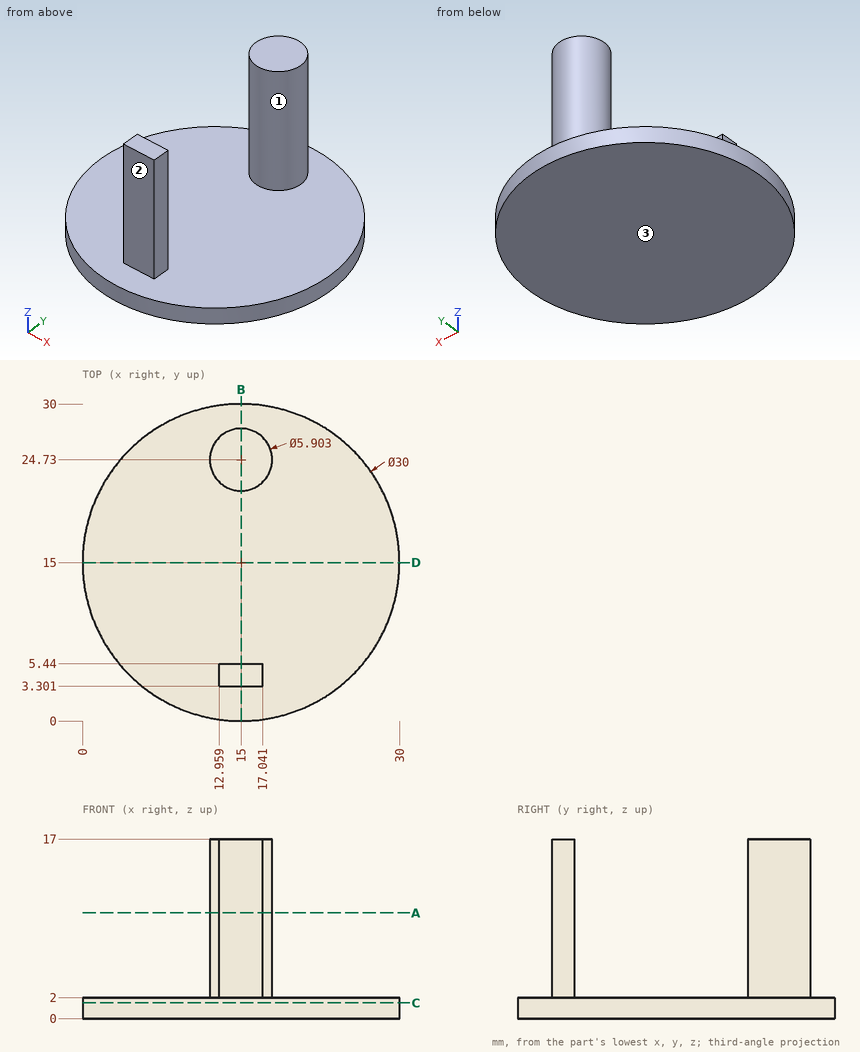
Input: dimensioned drawing with shaded views. Units: mm. Origin: part minimum x, y, z. Coordinates: 2 decimals unless noted, no trailing zeros. Loops run counter-clockwise (first coordinate to the right, second up) from the corner with the lowest first, then second, coordinate; pieces in that order, holes last.
Q1. Mould query, pull axis Y, two halves, no side actions, for the marked faces 1, 2 and 3. Classes: +Y half, -Y half, draft (parallel to the pull), parting line (faces both ways), or undercut.
Results are:
face 1: undercut
face 2: -Y half
face 3: draft
Q2. Section B-B, the plane x = 15. Return the cut outline in (y, z).
Results are:
outline: (0, 0) - (30, 0) - (30, 2) - (27.68, 2) - (27.68, 17) - (21.78, 17) - (21.78, 2) - (5.44, 2) - (5.44, 17) - (3.3, 17) - (3.3, 2) - (0, 2) - close
Q3. Contact query for flat-ended pins moving along their axis: pin 1 (8 mm diameter, centred on x = 27, y = 24, fed in from -Z); pin 2 (1.7 mm diameter, centred on y = 4, z = 10, fed in from +X); pin 3 (5 mm diameter, centred on x = 25.5, z = 3, fed in from -Y) (1 decimal); pin 4 (2 mm diameter, centred on x = 12.5, z = 13, fed in from +Y). Output: stop coordinate, or through.
Results are:
pin 1: stops at z = 0
pin 2: stops at x = 17.04
pin 3: stops at y = 2.4
pin 4: stops at y = 27.27
Q4. Section C-C, the plane z = 1.5. Return the cut outline in (x, y), and give its area (3 significant figures).
Results are:
outline: circle Ø30 at (15, 15)
area: 707 mm2
Q5. Line query: line 1 along Z through (x, y) = (16, 10); line 2 along X through (y, z) = (4.25, 10); line 3 along X through (y, z) = (27.25, 15.5) (1 decimal). Output: solid intervals per line, ascending.
Results are:
line 1: z = 0 to 2
line 2: x = 12.96 to 17.04
line 3: x = 13.5 to 16.5
Q6. Section A-A, the plane z = 10. Return the cut outline in (x, y).
Results are:
outline: circle Ø5.9 at (15, 24.73); (12.96, 3.3) - (17.04, 3.3) - (17.04, 5.44) - (12.96, 5.44) - close
Q7. Section D-D, the plane y = 15. Return the cut outline in (x, z), and give its area (3 significant figures).
Results are:
outline: (0, 0) - (30, 0) - (30, 2) - (0, 2) - close
area: 60.0 mm2
